Source: CAD feature listing. Evaluate the final solid. Frame: model axes, mm. Face numbers are marked on the shaded views. A direction names the side the tool comes from. Round coordinates to 2 decimals unless told otherwise and drop trailing zeros. Loops run counter-clockwise (first coordinate to the right, second up) from the corner with the lowest first, then second, coordinate; pieces in that order, holes last. Notation, with made-up numbers: M 9,-11 L 58,-11 A27 cw 58,6 Z; hole C 81,23 d5. An arc over 180 degrees is marked long. Answer as a JSON object with one key per item and string values.
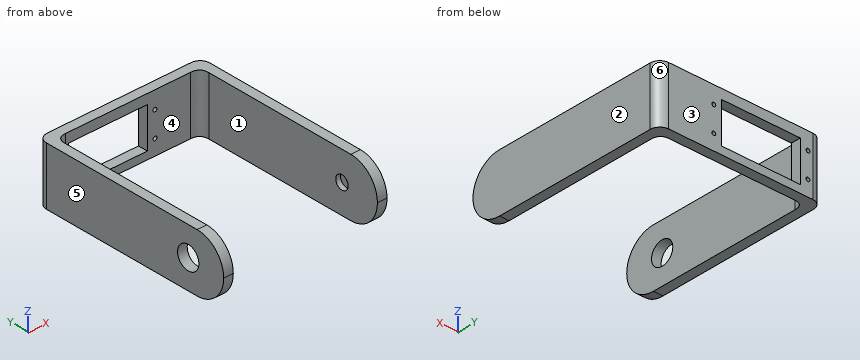
from build123d import *

# Parameters (mm, degrees)
F1_DEPTH    = 30
F3_START    = 37.5
F2_R        = 3.5
F3_DEPTH    = 2.5
F5_START    = -37.5
F4_R        = 6
F5_DEPTH    = 5
F6_R        = 14.99999
F7_R        = 5
F8_T1_DEPTH = 30
F10_START   = -33
F9_W        = 41
F9_H        = 21
F10_DEPTH   = 12
F12_START   = -35
F11_R       = 1
F12_DEPTH   = 10


# Not quite as in the source:
# - a fillet or chamfer that OpenCascade refuses, or shapes differently, is made with other operations: its cross-section is extruded or revolved along the edge and cut away or added
# - a fillet or chamfer is up to 0.001 mm smaller than in the source, because OpenCascade refuses the exact size


with BuildPart() as f1:
    # F0 (on Top) → F1 (new body)
    with BuildSketch(Plane.XY):
        Polygon((-42.5, -62.7966840421), (-37.5, -62.7966840421), (-37.5, 37.2033159579), (37.5, 37.2033159579), (37.5, -62.7966840421), (42.5, -62.7966840421), (42.5, 42.2033159579), (-42.5, 42.2033159579), align=None)
    extrude(amount=F1_DEPTH)

    # F2 (on Right) → F3 (cut)
    with BuildSketch(Plane.YZ.offset(F3_START)):
        with Locations((-42.7966840421, 15)):
            Circle(F2_R)
    extrude(amount=F3_DEPTH, mode=Mode.SUBTRACT)

    # F4 (on Right) → F5 (cut)
    with BuildSketch(Plane.YZ.offset(F5_START)):
        with Locations((-42.7966840421, 15)):
            Circle(F4_R)
    extrude(amount=-F5_DEPTH, mode=Mode.SUBTRACT)

    # F6 (radius 15 in the source; OpenCascade refuses exactly that, so slightly less here)
    f6_edges = [f1.edges().sort_by_distance(p)[0] for p in [
        (40, -62.796684, 30),
        (40, -62.796684, 0),
        (-40, -62.796684, 30),
        (-40, -62.796684, 0),
    ]]
    fillet(f6_edges, radius=F6_R)

    # F7
    f7_edges = [f1.edges().sort_by_distance(p)[0] for p in [
        (-42.5, 42.203316, 15),
        (42.5, 42.203316, 15),
    ]]
    fillet(f7_edges, radius=F7_R)

    # F8: fillet of radius 5 on 2 edges, made by hand

    # F8_s2 → F8_t1 (join)
    with BuildSketch(Plane.XY):
        with BuildLine():
            add(Edge.make_bspline(
                [(-37.5, 32.2033159579), (-37.5, 37.2033159579), (-32.5, 37.2033159579)],
                knots=[0, 0, 0, 1, 1, 1], degree=2, weights=[1, 1, 1]))
            Line((-32.5, 37.2033159579), (-37.5, 37.2033159579))
            Line((-37.5, 37.2033159579), (-37.5, 32.2033159579))
        make_face()
        with BuildLine():
            add(Edge.make_bspline(
                [(32.5, 37.2033159579), (37.5, 37.2033159579), (37.5, 32.2033159579)],
                knots=[0, 0, 0, 1, 1, 1], degree=2, weights=[1, 1, 1]))
            Line((37.5, 32.2033159579), (37.5, 37.2033159579))
            Line((37.5, 37.2033159579), (32.5, 37.2033159579))
        make_face()
    extrude(amount=F8_T1_DEPTH)

    # F9 (on Front) → F10 (cut)
    with BuildSketch(Plane.XZ.offset(F10_START)):
        with Locations((-10.5, 14.5)):
            Rectangle(F9_W, F9_H)
    extrude(amount=-F10_DEPTH, mode=Mode.SUBTRACT)

    # F11 (on Front) → F12 (cut)
    with BuildSketch(Plane.XZ.offset(F12_START)):
        with Locations((14, 21)):
            Circle(F11_R)
        with Locations((14, 8)):
            Circle(F11_R)
        with Locations((-35, 21)):
            Circle(F11_R)
        with Locations((-35, 8)):
            Circle(F11_R)
    extrude(amount=-F12_DEPTH, mode=Mode.SUBTRACT)


solid = f1.part
Item 1: Pull-direction query (X, two-part tool) for the marked faces 3, 4, 5 and 6; classes: pulls with the +X half, pulls with the -X half, needs draft (parallel to the pull), parting line crosses it, or undercut.
Answer sheet:
{"face 3": "needs draft", "face 4": "undercut", "face 5": "pulls with the -X half", "face 6": "pulls with the +X half"}
Item 2: Section B-B on y = -14.5. Return the cut outline in (x, z).
Answer sheet:
{"outline": "M -42.5,0 L -37.5,0 L -37.5,30 L -42.5,30 Z; M 37.5,0 L 42.5,0 L 42.5,30 L 37.5,30 Z"}
Item 3: Contact query for flat-ended pins moving along their axis: pin 1 Ø2.5 at (x, z) = (-35, 8) entering from -Y; pin 2 Ø11 at (y, z) = (-42.8, 15) entering from -X; pin 3 Ø2.5 at (x, z) = (14, 8) entering from +Y; pin 4 Ø2 at (y, z) = (-43.5, 16.5) entering from -X. Output: stop coordinate, or through.
Answer sheet:
{"pin 1": "stops at y = 35.95", "pin 2": "stops at x = 37.5", "pin 3": "stops at y = 42.2", "pin 4": "stops at x = 40"}
Item 4: Access query for the marked faces 1 and 2. Directions: +Z, -Z, +X, -X, +Y, -Y. A direction counts if a zero-diameter tool reaches every point of the face in a straight line with its end or side. Return the directions, or none.
Answer sheet:
{"face 1": "+Z, -Z, -Y", "face 2": "+Z, -Z, +X, +Y, -Y"}
Item 5: Section C-C on z = 16.5. Give the number of separate pieces and of enclosed holes in the cut face, then the cut area to 3 significant figures.
Answer sheet:
{"separate pieces": "3", "enclosed holes": "0", "area": "1,140 mm²"}
Item 6: Line query: probe 1 along Z at (x, y) = (-35, 37.5); probe 2 along X at (y, z) = (31, 24); probe 3 along Y at (x, z) = (-26, 28). Output: solid intervals per line, ascending. Write a range as from..to.
Answer sheet:
{"probe 1": "z = 0..7, 9..20, 22..30", "probe 2": "x = -42.5..-37.5, 37.5..42.5", "probe 3": "y = 37.2..42.2"}
Item 7: Section A-A on x = -13.5. Return the cut outline in (y, z).
Answer sheet:
{"outline": "M 37.2,0 L 42.2,0 L 42.2,4 L 37.2,4 Z; M 37.2,25 L 42.2,25 L 42.2,30 L 37.2,30 Z"}
